The listing builds one solid part. Answer for the finished solid, in the listing's coordinates (mm). A direction names the side the tool comes from. Give positions to 0.01 mm unless a question says otherwise; leave off trailing zeros. Loops run counter-clockwise (first coordinate to the right, second up) from the corner with the lowest first, then second, coordinate; pieces in that order, holes last.
Item 1: Section C-C, the plane y = 18 is taken. Give the vertices of the cut face in (x, z), and give its area (3 significant figures).
Item 2: Section A-A, the plane x = 25.25 is taken. Give the vertices of the cut face in (y, z).
Item 3: Section B-B, the plane z = 10 is taken. Give the vertices of the cut face in (x, y), and give its area (3 significant figures).
Item 4: Section D-D, the plane x = 17 is taken. Give the vertices of the cut face in (y, z).
Item 5: Consider line 1 along X through (y, z) = (27.8, 6.25); line 2 along Z through (x, y) = (25.25, 16.5); line 3 along X through (y, z) = (16.95, 6.25). Determine where each line is inside the solid, lowest interval first.
Item 6: The mould has two halves that part along X. Classify faces 1 (the face through (6, 30, 7.4)), 2 (the face through (-4.75, 17, 3)), 3 (the face through (24.25, 17.27, 6.22)): pulls with the +X half, pulls with the -X half, needs draft (parallel to the pull), parting line crosses it, or undercut.
Item 7: Each of these flat-tipped pins is pushed along its axis until it touches: pin 1 Ø1.4 at (x, z) = (26, 6.5) entering from +Y; pin 2 Ø3 at (y, z) = (7, 7) entering from -X; pin 3 Ø0.6 at (x, z) = (6, 6) entering from +Y; pin 4 Ø1.8 at (x, z) = (25.25, 6.25) entering from -Y. Where does it stop, or does it pass through?
Item 8: A tool of negligible diameter and unlimited length cuts with its end or side. For faces 4 (the face through (0.005, 24.972, 6.011)), 5 (the face through (27, 17, 7.05)), 6 (the face through (18, 23, 6)), from which of +Z, -Z, +X, -X, +Y, -Y can it reach the whole face along a straight path? Write none if from no direction.
from build123d import *

# Parameters (mm, degrees)
RESSALTO_EXTRUS_O1_DEPTH = 12.5
CORTE_EXTRUS_O1_DEPTH    = 36.616885041
ESBO_O3_R                = 6.25
ESBO_O3_R_2              = 2.5
RESSALTO_EXTRUS_O3_DEPTH = 4
ESBO_O4_R                = 2.5
ESBO_O4_R_2              = 1
RESSALTO_EXTRUS_O4_DEPTH = 3
RESSALTO_EXTRUS_O5_DEPTH = 3
PADR_OCIRCULAR1_COUNT    = 24


with BuildPart() as part:
    # Esboço1 → Ressalto-extrusão1 (new body)
    with BuildSketch(Plane.XY):
        Polygon((0, 0), (0, 16), (-4.75, 16), (-4.75, 18.5), (0, 18.5), (0, 23), (23, 23), (23, 18.5), (27.75, 18.5), (27.75, 16), (23, 16), (23, 0), align=None)
    extrude(amount=RESSALTO_EXTRUS_O1_DEPTH)

    # Esboço2 → Corte-extrusão1 (cut, through all)
    with BuildSketch(Plane(origin=(0, 18.5, 0), x_dir=(1, 0, 0), z_dir=(0, 1, 0))):
        with BuildLine():
            ThreePointArc((-2.85, -7.05), (-3.25, -6.25), (-2.85, -5.45))
            Line((-2.85, -5.45), (-4.75, -5.45))
            Line((-4.75, -5.45), (-4.75, -7.05))
            Line((-4.75, -7.05), (-2.85, -7.05))
        make_face()
        with BuildLine():
            ThreePointArc((-1.25, -6.25), (-1.802786405, -5.355572809), (-2.85, -5.45))
            Line((-2.85, -5.45), (-2.85, -7.05))
            ThreePointArc((-2.85, -7.05), (-1.802786405, -7.144427191), (-1.25, -6.25))
        make_face()
        with BuildLine():
            Line((-2.85, -7.05), (-2.85, -5.45))
            ThreePointArc((-2.85, -5.45), (-3.25, -6.25), (-2.85, -7.05))
        make_face()
        with BuildLine():
            ThreePointArc((26.25, -6.25), (26.144427191, -5.802786405), (25.85, -5.45))
            Line((25.85, -5.45), (25.85, -7.05))
            ThreePointArc((25.85, -7.05), (26.144427191, -6.697213595), (26.25, -6.25))
        make_face()
        with BuildLine():
            Line((25.85, -7.05), (25.85, -5.45))
            ThreePointArc((25.85, -5.45), (24.25, -6.25), (25.85, -7.05))
        make_face()
        with BuildLine():
            Line((27.75, -5.45), (25.85, -5.45))
            ThreePointArc((25.85, -5.45), (26.144427191, -5.802786405), (26.25, -6.25))
            ThreePointArc((26.25, -6.25), (26.144427191, -6.697213595), (25.85, -7.05))
            Line((25.85, -7.05), (27.75, -7.05))
            Line((27.75, -7.05), (27.75, -5.45))
        make_face()
    extrude(amount=-CORTE_EXTRUS_O1_DEPTH, mode=Mode.SUBTRACT)

    # Esboço3 → Ressalto-extrusão3 (add)
    with BuildSketch(Plane(origin=(0, 23, 0), x_dir=(1, 0, 0), z_dir=(0, 1, 0))):
        with BuildLine():
            ThreePointArc((12.137931034, -4.153629772), (12.789692169, -3.8530305), (13.5, -3.75))
            Line((13.5, -3.75), (11.978219619, -3.75))
            ThreePointArc((11.978219619, -3.75), (12.061580529, -3.95042792), (12.137931034, -4.153629772))
        make_face()
        with BuildLine():
            Line((11.978219619, -8.75), (13.5, -8.75))
            ThreePointArc((13.5, -8.75), (12.789692169, -8.6469695), (12.137931034, -8.346370228))
            ThreePointArc((12.137931034, -8.346370228), (12.061580529, -8.54957208), (11.978219619, -8.75))
        make_face()
        with BuildLine():
            ThreePointArc((12.137931034, -8.346370228), (12.789692169, -8.6469695), (13.5, -8.75))
            Line((13.5, -8.75), (13.5, -3.75))
            ThreePointArc((13.5, -3.75), (12.789692169, -3.8530305), (12.137931034, -4.153629772))
            ThreePointArc((12.137931034, -4.153629772), (12.408817621, -5.186296321), (12.5, -6.25))
            ThreePointArc((12.5, -6.25), (12.408817621, -7.313703679), (12.137931034, -8.346370228))
        make_face()
        with BuildLine():
            Line((13.5, -3.75), (13.5, -8.75))
            ThreePointArc((13.5, -8.75), (15.267766953, -8.017766953), (16, -6.25))
            ThreePointArc((16, -6.25), (15.267766953, -4.482233047), (13.5, -3.75))
        make_face()
        with Locations((6.25, -6.25)):
            Circle(ESBO_O3_R)
        with Locations((13.5, -6.25)):
            Circle(ESBO_O3_R_2)
        with BuildLine():
            Line((8.733610526, -8.75), (11.978219619, -8.75))
            ThreePointArc((11.978219619, -8.75), (12.061580529, -8.54957208), (12.137931034, -8.346370228))
            ThreePointArc((12.137931034, -8.346370228), (11, -6.25), (12.137931034, -4.153629772))
            ThreePointArc((12.137931034, -4.153629772), (12.061580529, -3.95042792), (11.978219619, -3.75))
            Line((11.978219619, -3.75), (8.733610526, -3.75))
            Line((8.733610526, -3.75), (8.733610526, -8.75))
        make_face()
        with BuildLine():
            ThreePointArc((11.978219619, -3.75), (0, -6.25), (11.978219619, -8.75))
            Line((11.978219619, -8.75), (8.733610526, -8.75))
            Line((8.733610526, -8.75), (8.733610526, -3.75))
            Line((8.733610526, -3.75), (11.978219619, -3.75))
        make_face()
    extrude(amount=RESSALTO_EXTRUS_O3_DEPTH)

    # Esboço4 → Ressalto-extrusão4 (add)
    with BuildSketch(Plane(origin=(0, 27, 0), x_dir=(1, 0, 0), z_dir=(0, 1, 0))):
        with Locations(Location((6.25, -6.25, 0), (0, 0, 270))):
            Circle(ESBO_O4_R)
        with Locations(Location((6.25, -6.25, 0), (0, 0, 270))):
            Circle(ESBO_O4_R_2, mode=Mode.SUBTRACT)
    extrude(amount=RESSALTO_EXTRUS_O4_DEPTH)

    # Esboço5 → Ressalto-extrusão5 (add)
    with BuildSketch(Plane(origin=(0, 30, 0), x_dir=(1, 0, 0), z_dir=(0, 1, 0))):
        with BuildLine():
            Line((5.952990595, -3.767705615), (6.103919204, -3.507984418))
            ThreePointArc((6.103919204, -3.507984418), (6.277405699, -3.408473433), (6.450327987, -3.508961652))
            Line((6.450327987, -3.508961652), (6.602949214, -3.77504003))
            Line((6.602949214, -3.77504003), (5.952990595, -3.767705615))
        make_face()
    ressalto_extrus_o5 = extrude(amount=-RESSALTO_EXTRUS_O5_DEPTH)

    # PadrãoCircular1: Ressalto-extrusão5 ×24 about axis
    padr_ocircular1_axis = Axis((6.25, 0, 6.25), (0, 1, 0))
    for i in range(1, PADR_OCIRCULAR1_COUNT):
        add(ressalto_extrus_o5.rotate(padr_ocircular1_axis, i * 360 / PADR_OCIRCULAR1_COUNT))


solid = part.part
Worked answers:
1. outline: (-4.75, 0) - (27.75, 0) - (27.75, 5.45) - (25.85, 5.45) arc R1 cw (long way) to (25.85, 7.05) - (27.75, 7.05) - (27.75, 12.5) - (-4.75, 12.5) - (-4.75, 7.05) - (-2.85, 7.05) arc R1 cw (long way) to (-2.85, 5.45) - (-4.75, 5.45) - close
1. area: 395 mm2
2. outline: (16, 0) - (18.5, 0) - (18.5, 5.25) - (16, 5.25) - close; (16, 7.25) - (18.5, 7.25) - (18.5, 12.5) - (16, 12.5) - close
3. outline: (-4.75, 16) - (0, 16) - (0, 0) - (23, 0) - (23, 16) - (27.75, 16) - (27.75, 18.5) - (23, 18.5) - (23, 23) - (11.25, 23) - (11.25, 27) - (1.25, 27) - (1.25, 23) - (0, 23) - (0, 18.5) - (-4.75, 18.5) - close
3. area: 593 mm2
4. outline: (0, 0) - (23, 0) - (23, 12.5) - (0, 12.5) - close
5. line 1: x = 3.41 to 5.25, 7.25 to 9.09
5. line 2: z = 0 to 5.25, 7.25 to 12.5
5. line 3: x = -1.25 to 24.25
6. face 1: needs draft
6. face 2: pulls with the -X half
6. face 3: undercut
7. pin 1: stops at y = 18.5
7. pin 2: stops at x = 0
7. pin 3: stops at y = 27
7. pin 4: passes through
8. face 4: +Y
8. face 5: +X, +Y, -Y
8. face 6: +X, +Y
